Autodesk Inventor part; units mm, degrees
sketch "Skizze1" plane through (0, 0, 0) normal (0, 1, 0) x (-1, 0, 0)
  line L0 (-55, 0) -> (-55, -55)
  line L1 (-55, -55) -> (-35.3027, -161.5294)
  line L2 (0, 0) -> (-55, 0)
  line L3 (79.5383, 0) -> (-92.2301, 0)
  line L4 (-36.5551, -163.7611) -> (-60.3632, -172.8644)
  line L5 (-60.3632, -178.4687) -> (-35, -188.1665)
  line L6 (-35, -188.1665) -> (-30, -188.1665)
  line L7 (-30, -188.1665) -> (-30, -200.1665)
  line L8 (-30, -200.1665) -> (-30, -200.1665)
  line L9 (-36, -206.1665) -> (-36, -206.1665)
  line L10 (-36, -206.1665) -> (-36, -206.1665)
  line L11 (-44, -214.1665) -> (-44, -214.1665)
  line L12 (-44, -214.1665) -> (-61, -214.1665)
  line L13 (-61, -214.1665) -> (-61, -214.1665)
  line L14 (-47, -228.1665) -> (-47, -228.1665)
  line L15 (-47, -228.1665) -> (0, -228.1665)
  arc A0 (-61, -214.1665) -> (-47, -228.1665) centre (-47, -214.1665) ccw
  arc A1 (-44, -214.1665) -> (-36, -206.1665) centre (-44, -206.1665) ccw
  arc A2 (-30, -200.1665) -> (-36, -206.1665) centre (-30, -206.1665) ccw
  arc A3 (-60.3632, -172.8644) -> (-60.3632, -178.4687) centre (-59.2917, -175.6665) ccw
  arc A4 (-36.5551, -163.7611) -> (-35.3027, -161.5294) centre (-37.2694, -161.893) ccw
  line L16 (0, 0) -> (0, -228.1665)
  point P0 (-35, -163.1665)
  point P1 (-67.6917, -175.6665)
  point P2 (-36, -200.1665)
  point P3 (-36, -214.1665)
  point P4 (-61, -228.1665)
  dimension "d1" = 55
  dimension "d54" = 110
  dimension "d55" = 55
  dimension "d56" = 20
  dimension "d57" = 35
  dimension "d58" = 35
  dimension "d59" = 25
  dimension "d60" = 12.5
  dimension "d61" = 5
  dimension "d62" = 12
  dimension "d63" = 6
  dimension "d64" = 6
  dimension "d65" = 8
  dimension "d66" = 8
  dimension "d67" = 17
  dimension "d68" = 14
  dimension "d69" = 14
  dimension "d70" = 47
  dimension "d71" = 14
  dimension "d72" = 8
  dimension "d73" = 6
  dimension "d74" = 3
  dimension "d75" = 2
extrude "Extrusion1" add sketch "Skizze1" along normal blind 1.5
mirror "Spiegeln1" about plane through (0, 0, 0) normal (1, 0, 0) of "Extrusion1"
sketch "Skizze2" plane through (0, 1.5, 0) normal (0, 1, 0) x (1, 0, 0)
  line L0 (55, 0) -> (-55, 0)
  line L1 (-55, 0) -> (-55, 55)
  line L2 (55, 0) -> (55, 55)
  arc A0 (60.3632, 172.8644) -> (60.3632, 178.4687) centre (59.2917, 175.6665) ccw
  line L3 (47, 228.1665) -> (-47, 228.1665)
  point P0 (0, 0)
  point P1 (-32, 60)
  point P2 (32, 60)
  point P3 (-32, 130)
  point P4 (32, 130)
  point P5 (33.5, 150)
  point P6 (33.5, 160)
  point P7 (-8.8, 160)
  point P8 (-8.8, 150)
  point P9 (45, 170)
  point P10 (45, 182)
  point P11 (0, 221.1665)
  point P12 (37, 221.1665)
  point P13 (-37, 221.1665)
  point P14 (-45, 182)
  point P15 (-45, 170)
  dimension "d78" = 60
  dimension "d79" = 23
  dimension "d80" = 60
  dimension "d81" = 23
  dimension "d82" = 70
  dimension "d83" = 70
  dimension "d84" = 23
  dimension "d85" = 23
  dimension "d86" = 20
  dimension "d87" = 1.5
  dimension "d88" = 10
  dimension "d89" = 1.5
  dimension "d91" = 20
  dimension "d92" = 10
  dimension "d93" = 42.3
  dimension "d94" = 42.3
  dimension "d95" = 13
  dimension "d97" = 10
  dimension "d98" = 13
  dimension "d99" = 12
  dimension "d100" = 7
  dimension "d101" = 7
  dimension "d102" = 7
  dimension "d103" = 10
  dimension "d104" = 37
  dimension "d105" = 37
  dimension "d106" = 10
  dimension "d107" = 12
  dimension "d108" = 40
  dimension "d109" = 13
  dimension "d110" = 13
hole "Bohrung1" at (-32, 1.5, -60) at (32, 1.5, -60) at (-32, 1.5, -130) at (32, 1.5, -130) at (33.5, 1.5, -150) at (33.5, 1.5, -160) at (-8.8, 1.5, -160) at (-8.8, 1.5, -150) at (45, 1.5, -170) at (45, 1.5, -182) at (0, 1.5, -221.1665) at (37, 1.5, -221.1665) at (-37, 1.5, -221.1665) at (-45, 1.5, -182) at (-45, 1.5, -170) direction (0, -1, 0) diameter 3 end through all
sketch "Skizze4" plane through (55, 0, 0) normal (1, 0, 0) x (0, 0, -1)
  line L0 (0, 1.5) -> (55, 1.5)
  line L1 (5, 1.5) -> (45, 1.5)
  line L2 (45, 1.5) -> (45, 0)
  line L3 (45, 0) -> (5, 0)
  line L4 (0, 0) -> (55, 0)
  line L5 (5, 1.5) -> (5, 0)
  line L6 (0, 0) -> (0, 1.5)
  dimension "d121" = 40
  dimension "d122" = 5
  dimension "d123" = 40
extrude "Extrusion2" add sketch "Skizze4" along normal blind 3 contours L0 L2 L3 L5
sketch "Skizze5" plane through (0, 1.5, 0) normal (0, 1, 0) x (1, 0, 0)
  line L0 (55, 5) -> (58, 5)
  line L1 (56.5, 5) -> (56.5, 45)
  line L2 (55, 45) -> (58, 45)
  line L3 (58, 45) -> (58, 5)
  line L4 (58, 5) -> (56.5, 5)
  line L5 (56.5, 45) -> (58, 45)
  point P0 (0, 0)
  dimension "d126" = 1.5
extrude "Extrusion3" add sketch "Skizze5" along normal blind 40
fillet "Rundung1" radius 2 1 edges at (58, 0, -25)
fillet "Rundung2" radius 20 2 edges at (57.25, 41.5, -5) (57.25, 41.5, -45)
mirror "Spiegeln2" about plane through (0, 0, 0) normal (1, 0, 0) of "Extrusion2", "Extrusion3"
mirror "Spiegeln3" about plane through (0, 0, 0) normal (1, 0, 0) of "Rundung2"
sketch "Skizze6" plane through (58, 0, 0) normal (1, 0, 0) x (0, 0, -1)
  arc A0 (18.5, 15) -> (31.5, 15) centre (25, 15) ccw
  arc A1 (31.5, 28.5) -> (18.5, 28.5) centre (25, 28.5) ccw
  line L0 (5, 2) -> (5, 21.5)
  line L1 (45, 2) -> (5, 2)
  line L2 (18.5, 28.5) -> (18.5, 15)
  line L3 (31.5, 28.5) -> (31.5, 15)
  line L4 (45, 1.5) -> (55, 1.5)
  point P0 (0, 0)
  dimension "d131" = 13
  dimension "d132" = 13
  dimension "d133" = 20
  dimension "d135" = 20
  dimension "d136" = 13.5
  dimension "d143" = 13.5
extrude "Extrusion4" cut sketch "Skizze6" against normal blind 1.5
sketch "Skizze7" plane through (58, 0, 0) normal (1, 0, 0) x (0, 0, -1)
  line L0 (0, 1.5) -> (5, 1.5)
  line L1 (45, 1.5) -> (55, 1.5)
  line L2 (5, 2) -> (5, 21.5)
  line L3 (45, 2) -> (45, 21.5)
  line L4 (45, 2) -> (5, 2)
  line L5 (18.5, 15) -> (18.5, 28.5)
  arc A0 (18.5, 15) -> (31.5, 15) centre (25, 15) ccw
  point P0 (0, 0)
  point P1 (10, 21.5)
  dimension "d146" = 20
  dimension "d147" = 5
sketch "Skizze8" plane through (58, 0, 0) normal (1, 0, 0) x (0, 0, -1)
  line L0 (18.5, 15) -> (18.5, 28.5)
  arc A0 (18.5, 15) -> (31.5, 15) centre (25, 15) ccw
  point P0 (0, 0)
  point P1 (25, 21.5)
  dimension "d150" = 6.5
  dimension "d151" = 6.5
hole "Bohrung2" at (58, 21.5, -10) direction (-1, 0, 0) diameter 3 end through all
pattern_circular "Runde Anordnung1" count 6 over 360 about axis through (58, 21.5, -25) along (1, 0, 0) of "Bohrung2"
mirror "Spiegeln4" about plane through (0, 0, 0) normal (1, 0, 0) of "Extrusion4"
ref_plane "Arbeitsebene1" through (0, 0, 0) normal (1, 0, 0) x (0, 1, 0)
properties part number "grundplatte"
Could you check a few things on this model? Use its own coordinates, in mm. A direction names the side the tool comes from. Round coordinates to 2 decimals unless told otherwise and drop trailing zeros. Loops run counter-clockwise (first coordinate to the right, second up) from the corner with the lowest first, then second, coordinate; pieces in that order, holes last. Notation, with made-up numbers: (83.5, -36) -> (132.5, -36) arc R16 ccw to (132.5, -23) -> close; hole circle Ø2 at (42.5, -27). An arc over 180 degrees is marked (long way). Put each result on its own line as item: value.
Q1. I want a section at A-A on x = 21.5. Write out the boundary of the cut face in (y, z), and give its area (3 significant figures).
Checks:
outline: (0, -228.17) -> (1.5, -228.17) -> (1.5, 0) -> (0, 0) -> close
area: 342 mm2
Q2. Please list where these lines run through material, in increasing order: line 1 (Z direction, x = 57, y = 21); line 2 (X direction, y = 0.6, z = -150); line 3 (Y direction, x = 25, z = -67.5). Write a range as from..to.
Checks:
line 1: -45..-41.41, -38.59..-31.5, -18.5..-11.41, -8.59..-5
line 2: -37.43..-10.3, -7.3..32, 35..37.43
line 3: 0..1.5
Q3. Thinking about a two-plate mould opening in Z: for faces 1 (the flat face through (47.86, 0.74, -183.25)), 2 (the cylindrical face through (56.79, 0.74, -224.174)), 3 (the flat face through (1, 1.5, -87)), which applies, pulls with the +Z half, pulls with the -Z half, needs draft (parallel to the pull), parting line crosses it, or undercut?
Checks:
face 1: undercut
face 2: pulls with the -Z half
face 3: needs draft
Q4. For pin 1 Ø1.6 at (x, y) = (-57, 22) entering from +Z; pin 2 Ø6 at (x, z) = (-25.5, -151) entering from +Y; pin 3 Ø1.6 at (y, z) = (0.5, -197) entering from -X; pin 4 Ø2.5 at (y, z) = (8.51, -32.5) entering from +X, each with a flat end and sliding along its axis, tell me the tip position at first contact or that it passes through.
Checks:
pin 1: z = -5
pin 2: y = 1.5
pin 3: x = -30
pin 4: through
Q5. Which directions (+Z, -Z, +X, -X, +Y, -Y) give clear straight access to the entire face, cutting with the end or side of a thin tool? Please do faces 4 (the flat face through (56.5, 21, -34)), 5 (the flat face through (-47.504, 0.74, -183.385)), 6 (the cylindrical face through (34.29, 0.74, -201.97)).
Checks:
face 4: +Z, -Z, +Y
face 5: -X, +Y, -Y
face 6: +X, +Y, -Y
